Source: CAD feature listing. Evaluate the final solid. Frame: model axes, mm. Give positions to 0.01 mm unless a question says otherwise; leave off trailing zeros. Write each loop counter-clockwise with the first axis right and the second up, starting at its lowest first coordinate (ties: lowest second). Pieces come first, ordered by that corner, then holes. Notation, with made-up numbers: (87.25, -8.75) -> (126.25, -8.75) arc R21 ccw to (126.25, 14.25) -> close; hole circle Ø7 at (-11.5, 66.5). An arc over 180 degrees is marked (long way). Use one line per item in the form item = value. Start each with the question number.
(1) Draft query along Y for faces 1 (the face through (-24.89, -32.83, 2.54)), 2 (the face through (1.429, 41.325, 2.465)), 3 (the face through (-19, 21, 0)), 4 (the face through (28.34, -25.8, 2.54)). Return one class per face: pulls with the +Y half, pulls with the -Y half, needs draft (parallel to the pull), parting line crosses it, or undercut.
(2) Cut plane D-D, the plane y = -4.5. Output: boundary loops of the cut face in (x, z), and give its area (3 significant figures).
(3) Cut plane C-C, the plane z = 2. Count the separate pieces of the cut face and the enclosed holes in it, and give its area (3 significant figures).
(4) First-contact query: P1, Ø6.5, axis at x = 26.41, y = -26.41, coming from the +Z side; P2, Ø3, axis at y = 16, z = 3.5, coming from the -X side. Flat tips, straight axial feed; report the tip coordinate or a pass-through.
(5) Cut plane A-A, the plane x = 0. Output: boundary loops of the cut face in (y, z) (3 decimals).
(6) Material intervals for line 1 along Y through (x, z) = (0, 3.7) (3 decimals); line 2 along X through (y, z) = (-14, 3.05); line 3 along Y through (x, z) = (-37.35, 1.45) (3 decimals), sorted ascending. Write a range as from..to.
(7) Cut plane B-B, the plane x = -12. Output: boundary loops of the cut face in (y, z).
from build123d import *

# Parameters (mm, degrees)
SKETCH_1_R          = 41.35
SKETCH_1_R_2        = 2.025
SKETCH_1_R_3        = 25
EXTRUDE_1_DEPTH     = 5
SKETCH_2_R          = 2.025
CUT_EXTRUDE_1_DEPTH = 5
CUT_EXTRUDE_START   = -5
CUT_EXTRUDE_2_DEPTH = 5
FILLET_1_R          = 3


with BuildPart() as part:
    # 草图1 → 凸台-拉伸1 (new body)
    with BuildSketch(Plane.XY):
        Circle(SKETCH_1_R)
        with Locations((0, 29)):
            Circle(SKETCH_1_R_2, mode=Mode.SUBTRACT)
        with Locations((25.11473671, 14.5)):
            Circle(SKETCH_1_R_2, mode=Mode.SUBTRACT)
        with Locations((25.11473671, -14.5)):
            Circle(SKETCH_1_R_2, mode=Mode.SUBTRACT)
        with Locations((0, -29)):
            Circle(SKETCH_1_R_2, mode=Mode.SUBTRACT)
        with Locations((-25.11473671, -14.5)):
            Circle(SKETCH_1_R_2, mode=Mode.SUBTRACT)
        with Locations((-25.11473671, 14.5)):
            Circle(SKETCH_1_R_2, mode=Mode.SUBTRACT)
        Circle(SKETCH_1_R_3, mode=Mode.SUBTRACT)
    extrude(amount=EXTRUDE_1_DEPTH)

    # 草图2 → 切除-拉伸1 (cut)
    with BuildSketch(Plane.XY.offset(5)):
        with Locations((0, 37.35)):
            Circle(SKETCH_2_R)
        with Locations((26.410438277, 26.410438277)):
            Circle(SKETCH_2_R)
        with Locations((37.35, 0)):
            Circle(SKETCH_2_R)
        with Locations((26.410438277, -26.410438277)):
            Circle(SKETCH_2_R)
        with Locations((0, -37.35)):
            Circle(SKETCH_2_R)
        with Locations((-26.410438277, -26.410438277)):
            Circle(SKETCH_2_R)
        with Locations((-37.35, 0)):
            Circle(SKETCH_2_R)
        with Locations((-26.410438277, 26.410438277)):
            Circle(SKETCH_2_R)
    extrude(amount=-CUT_EXTRUDE_1_DEPTH, mode=Mode.SUBTRACT)

    # 草图3 → 切除-拉伸2 (cut)
    with BuildSketch(Plane.XY.offset(5).offset(CUT_EXTRUDE_START)):
        with BuildLine():
            Line((-24.916309919, -33), (24.916309919, -33))
            ThreePointArc((24.916309919, -33), (0, -41.35), (-24.916309919, -33))
        make_face()
    extrude(amount=CUT_EXTRUDE_2_DEPTH, mode=Mode.SUBTRACT)

    # 圆角1
    fillet_1_edges = [part.edges().sort_by_distance(p)[0] for p in [
        (24.916309919, -33, 2.5),
        (-24.916309919, -33, 2.5),
    ]]
    fillet(fillet_1_edges, radius=FILLET_1_R)


solid = part.part
Geometry says:
q1.face_1 = pulls with the -Y half
q1.face_2 = parting line crosses it
q1.face_3 = needs draft
q1.face_4 = undercut
q2.outline = (-41.1, 0) -> (-24.59, 0) -> (-24.59, 5) -> (-41.1, 5) -> close; (24.59, 0) -> (41.1, 0) -> (41.1, 5) -> (24.59, 5) -> close
q2.area = 165 mm^2
q3.separate_pieces = 1
q3.enclosed_holes = 14
q3.area = 2,960 mm^2
q4.P1 = 5
q4.P2 = -38.72
q5.outline = (-33, 0) -> (-31.025, 0) -> (-31.025, 5) -> (-33, 5) -> close; (-26.975, 0) -> (-25, 0) -> (-25, 5) -> (-26.975, 5) -> close; (25, 0) -> (26.975, 0) -> (26.975, 5) -> (25, 5) -> close; (31.025, 0) -> (35.325, 0) -> (35.325, 5) -> (31.025, 5) -> close; (39.375, 0) -> (41.35, 0) -> (41.35, 5) -> (39.375, 5) -> close
q6.line_1 = -33..-31.025, -26.975..-25, 25..26.975, 31.025..35.325, 39.375..41.35
q6.line_2 = -38.91..-27.08, -23.15..-20.71, 20.71..23.15, 27.08..38.91
q6.line_3 = -17.743..-2.025, 2.025..17.743
q7.outline = (-33, 0) -> (-21.93, 0) -> (-21.93, 5) -> (-33, 5) -> close; (21.93, 0) -> (39.57, 0) -> (39.57, 5) -> (21.93, 5) -> close
